```python
from build123d import *

# Parameters (mm, degrees)
EXTRU_MINCE1_DEPTH           = 21
ESQUISSE4_R                  = 4.9999999999999964
BOSS_EXTRU_2_DEPTH           = 21
ENL_V_MAT_EXTRU_2_DEPTH      = 79.88123984826811
ENL_V_MAT_EXTRU_2_DEPTH_BACK = 79.88123984826811
ESQUISSE5_R                  = 2.250000000000002
ENL_V_START                  = -7
ESQUISSE6_R                  = 4.9999999999999964
ENL_V_MAT_EXTRU_3_DEPTH      = 7
CONG_4_R                     = 3
CONG_6_R                     = 2.5
BOSS_EXTRU_3_START           = -21
BOSS_EXTRU_3_DEPTH           = 21
ENL_V_MAT_EXTRU_4_DEPTH      = 79.88123984826811
ENL_V_MAT_EXTRU_4_DEPTH_BACK = 79.88123984826811
ESQUISSE8_R                  = 1.7500000000000038


# Some blends are built 0.0001 mm under size
with BuildPart() as part:
    # Esquisse1 → Extru.-Mince1 (new body)
    with BuildSketch(Plane.XY):
        with BuildLine():
            ThreePointArc((52.49999999999999, 4.2e-16), (26.249999999999886, 45.46633369868308), (-26.250000000000224, 45.4663336986829))
            Line((-26.250000000000224, 45.4663336986829), (-23.750000000000203, 41.13620667976072))
            ThreePointArc((-23.750000000000203, 41.13620667976072), (23.749999999999897, 41.13620667976088), (47.49999999999999, -4.2e-16))
            Line((47.49999999999999, -4.2e-16), (52.49999999999999, 4.2e-16))
        make_face()
    extrude(amount=EXTRU_MINCE1_DEPTH)

    # Esquisse4 → Boss.-Extru.2 (add)
    with BuildSketch(Plane.XY.offset(21)):
        with Locations((50, 0)):
            Circle(ESQUISSE4_R)
    extrude(amount=-BOSS_EXTRU_2_DEPTH)

    # Esquisse5 → Enlèv. mat.-Extru.2 (cut, two sides: drawn at the far end of the back side and taken through both)
    with BuildSketch(Plane.XY.offset(21).offset(-ENL_V_MAT_EXTRU_2_DEPTH_BACK)):
        with Locations((50, 0)):
            Circle(ESQUISSE5_R)
    extrude(amount=ENL_V_MAT_EXTRU_2_DEPTH + ENL_V_MAT_EXTRU_2_DEPTH_BACK, mode=Mode.SUBTRACT)

    # Esquisse6 → Enlèv. mat.-Extru.3 (cut)
    with BuildSketch(Plane.XY.offset(21).offset(ENL_V_START)):
        with Locations((50, 0)):
            Circle(ESQUISSE6_R)
    extrude(amount=-ENL_V_MAT_EXTRU_3_DEPTH, mode=Mode.SUBTRACT)

    # Congé4
    # the kernel refuses this fillet: 3 mm, written as the material it adds along each edge
    with BuildSketch(Plane(origin=(47.3125, 4.216318743880709, 21), x_dir=(-0.7695454862891271, -0.6385920016192113, 0), z_dir=(0, 0, -1)), Plane(origin=(47.3125, 4.216318743880709, 7), x_dir=(-0.7695454862891271, -0.6385920016192113, 0), z_dir=(0, 0, -1))) as cong_4_piece_1:
        with BuildLine():
            CenterArc((1.6233202224653038, 2.976519037476766), CONG_4_R, 212.62585704290902, 50.20084903739968)
            ThreePointArc((-0.903307284750997, 1.359066274711204), (-0.45749046797105886, 0.6756536745373425), (0, 0))
            ThreePointArc((0, 0), (0.6243539317174114, 0.03913493753872468), (1.2487078634348219, 4e-17))
        make_face()
    extrude(amount=7)
    with BuildSketch(Plane(origin=(52.3125, 4.433096406576334, 21), x_dir=(0.8303156074241137, -0.5572934523820687, 0), z_dir=(0, 0, -1)), Plane(origin=(52.3125, 4.433096406576334, 7), x_dir=(0.8303156074241137, -0.5572934523820687, 0), z_dir=(0, 0, -1))) as cong_4_piece_2:
        with BuildLine():
            CenterArc((1.4311199733874571, -2.981766146537774), CONG_4_R, 96.3202818650538, 43.48897964287826)
            ThreePointArc((-0.8605810852935136, -1.0457634973555643), (-0.4269182279533879, -0.5256568983613493), (0, 0))
            ThreePointArc((0, 0), (0.5504307589951836, -0.03038975577037968), (1.100861517990363, 3e-17))
        make_face()
    extrude(amount=7)

    # Congé6
    cong_6_edges = [part.edges().sort_by_distance(p)[0] for p in [
        (-26.25000000000022, 45.46633369868291, 10.5),
        (-23.750000000000203, 41.13620667976072, 10.5),
    ]]
    fillet(cong_6_edges, radius=CONG_6_R - 0.0001)  # a hair under: the kernel refuses the full size

    # Esquisse7 → Boss.-Extru.3 (add)
    with BuildSketch(Plane.XY.offset(21).offset(BOSS_EXTRU_3_START)):
        with BuildLine():
            ThreePointArc((47.82358383341308, 21.659982209792123), (53.09263307440395, 19.324138097899965), (50.5577588361061, 14.147898129055626))
            ThreePointArc((50.5577588361061, 14.147898129055626), (49.33386259126014, 17.956057524597252), (47.82358383341308, 21.659982209792123))
        make_face()
    extrude(amount=BOSS_EXTRU_3_DEPTH)

    # Esquisse8 → Enlèv. mat.-Extru.4 (cut, two sides: drawn at the far end of the back side and taken through both)
    with BuildSketch(Plane.XY.offset(21).offset(-ENL_V_MAT_EXTRU_4_DEPTH_BACK)):
        with Locations((49.333862591260306, 17.956057524597313)):
            Circle(ESQUISSE8_R)
    extrude(amount=ENL_V_MAT_EXTRU_4_DEPTH + ENL_V_MAT_EXTRU_4_DEPTH_BACK, mode=Mode.SUBTRACT)


solid = part.part
```
The model under review builds one solid part; all positions refer to its coordinate system, in mm. A direction names the side the tool comes from. Round coordinates to 2 decimals unless told otherwise and drop trailing zeros. Order: outer loops, then holes, each group sorted by start corner. A loop starts at its lowest first (then second) coordinate and runs counter-clockwise, first axis right, second up.
Item 1: Machinability: for faces 5 (the cylindrical face through (52.52, 4.69, 17.55)), 6 (the cylindrical face through (47.02, 4.56, 17.55)), which of the approach directions +Z, -Z, +X, -X, +Y, -Y give a long, thin tool a straight path to every point of the face, cutting with its end or side? Answer none if there is none.
Working result:
face 5: +Z, -Z, +X
face 6: +Z, -Z, -X
Item 2: Add section C-C, the plane x = -15. State the section outline as (y, z) points.
Working result:
outline: (45.07, 0) - (50.31, 0) - (50.31, 21) - (45.07, 21) - close
Item 3: Add section B-B, the plane z = 2.5. Count the separate pieces of the cut face and the enclosed holes in it, and give its area (3 significant figures).
Working result:
separate pieces: 1
enclosed holes: 2
area: 576 mm2
Item 4: Add section A-A, the plane y = 0. State the section outline as (x, z) points.
Working result:
outline: (45, 0) - (47.75, 0) - (47.75, 7) - (45, 7) - close; (45, 14) - (47.75, 14) - (47.75, 21) - (45, 21) - close; (52.25, 0) - (55, 0) - (55, 7) - (52.25, 7) - close; (52.25, 14) - (55, 14) - (55, 21) - (52.25, 21) - close
Item 5: Draft analysis for pull direction Z (two halves, no side actions). For faces 1 (the flat face through (30, 39, 0)), 2 (the flat face through (27, 40, 21)), 3 (the flat face through (47.7, -0.9, 14)), 4 (the cylindrical face through (52.52, 4.69, 3.55)), state which applies: released by +Z, released by -Z, zero draft, split by the parting line, or undercut.
Working result:
face 1: released by -Z
face 2: released by +Z
face 3: undercut
face 4: zero draft
Item 6: Add section D-D, the plane y = 33. State the section outline as (x, z) points, and give its area (3 significant figures).
Working result:
outline: (34.17, 0) - (40.83, 0) - (40.83, 21) - (34.17, 21) - close
area: 140 mm2
Item 7: To check wall thickness, follow probe 1 along X at (y, z) = (0, 19); probe 2 along Y at (x, z) = (50, 18); probe 3 along X at (y, z) = (-1, 17.5). State the ranges of each line that lie inside material, in increasing order.
Working result:
probe 1: x = 45 to 47.75, 52.25 to 55
probe 2: y = -5 to -2.25, 2.25 to 16.34, 19.57 to 21.9
probe 3: x = 45.1 to 47.98, 52.02 to 54.9
Item 8: For pin 1 (6 mm diameter, centred on x = 2, z = 8, fed in from -Y); pin 2 (10 mm diameter, centred on x = 14, z = 15.5, fed in from -Y); pin 3 (12 mm diameter, centred on y = 17, z = 17.5, fed in from -X), all flat-tipped, find the tip position at first contact; note any pin that passes through.
Working result:
pin 1: stops at y = 47.24
pin 2: stops at y = 43.53
pin 3: stops at x = 41.56
